Could you check a few things on this drawing? It's one solid part, dimensions in mm from its lowest x, y, z. A direction names the side the tool comes from. Give positions to 0.01 mm unless a question says otherwise; leave off trailing zeros. Order: outer loops, then holes, each group sorted by start corner. A loop starts at its lowest first (then second) coordinate and runs counter-clockwise, first axis right, second up.
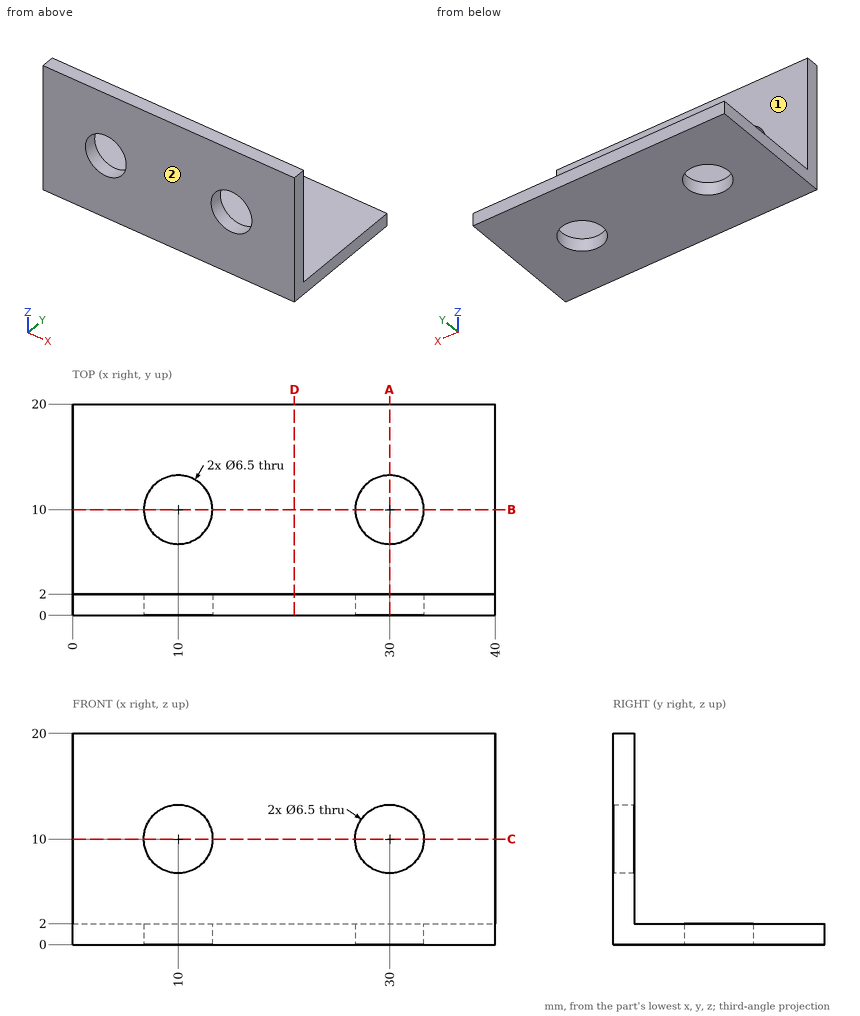
1) Suppose I cut it at D-D (x = 21). Please give me the cut outline in (y, z).
2) Which directions (+Z, -Z, +X, -X, +Y, -Y) give clear straight access to the entire face, cutting with the end or side of a thin tool? Please do the marked faces 1 and 2.
3) Suppose I cut it at A-A (x = 30). Please give me the cut outline in (y, z), and give its area (3 significant figures).
4) If I drill on line 1 (X direction, y = 1.4, z = 10); line 2 (Y direction, x = 10, z = 0.4); line 3 (Z direction, x = 19.5, y = 6.5), over which ranges is the centre line in solid material (lowest first)?
5) I'm going to push flat-ended pins straight in: pin 1 Ø10.5 at (x, y) = (30, 10) entering from +Z; pin 2 Ø8 at (x, z) = (16.5, 17) entering from +Y. Where does each tip first touch, or does it pass through?
6) Suppose I cut it at B-B (y = 10). Please give me the cut outline in (x, z).
Results:
1. outline: (0, 0) - (20, 0) - (20, 2) - (2, 2) - (2, 20) - (0, 20) - close
2. face 1: +Z, +X, -X, +Y
2. face 2: +Z, -Z, +X, -X, -Y
3. outline: (0, 0) - (6.75, 0) - (6.75, 2) - (2, 2) - (2, 6.75) - (0, 6.75) - close; (0, 13.25) - (2, 13.25) - (2, 20) - (0, 20) - close; (13.25, 0) - (20, 0) - (20, 2) - (13.25, 2) - close
3. area: 50.0 mm2
4. line 1: x = 0 to 6.75, 13.25 to 26.75, 33.25 to 40
4. line 2: y = 0 to 6.75, 13.25 to 20
4. line 3: z = 0 to 2
5. pin 1: stops at z = 2
5. pin 2: stops at y = 2
6. outline: (0, 0) - (6.75, 0) - (6.75, 2) - (0, 2) - close; (13.25, 0) - (26.75, 0) - (26.75, 2) - (13.25, 2) - close; (33.25, 0) - (40, 0) - (40, 2) - (33.25, 2) - close
